Geometry check sheet. Reference: drawing and pictorial views, mm from the part's lowest x, y, z. Round coordinates to 2 decimals unless told otherwise and drop trailing zeros. Loops run counter-clockwise (first coordinate to the right, second up) from the corner with the lowest first, then second, coordinate; pieces in that order, holes last. Notation, with made-up numbers: (45, -17) - (101, -17) arc R22 ccw to (101, 0) - close; hole circle Ø5 at (49.25, 59). An arc over 180 degrees is marked (long way). Return JSON: item names as keys, results as strings.
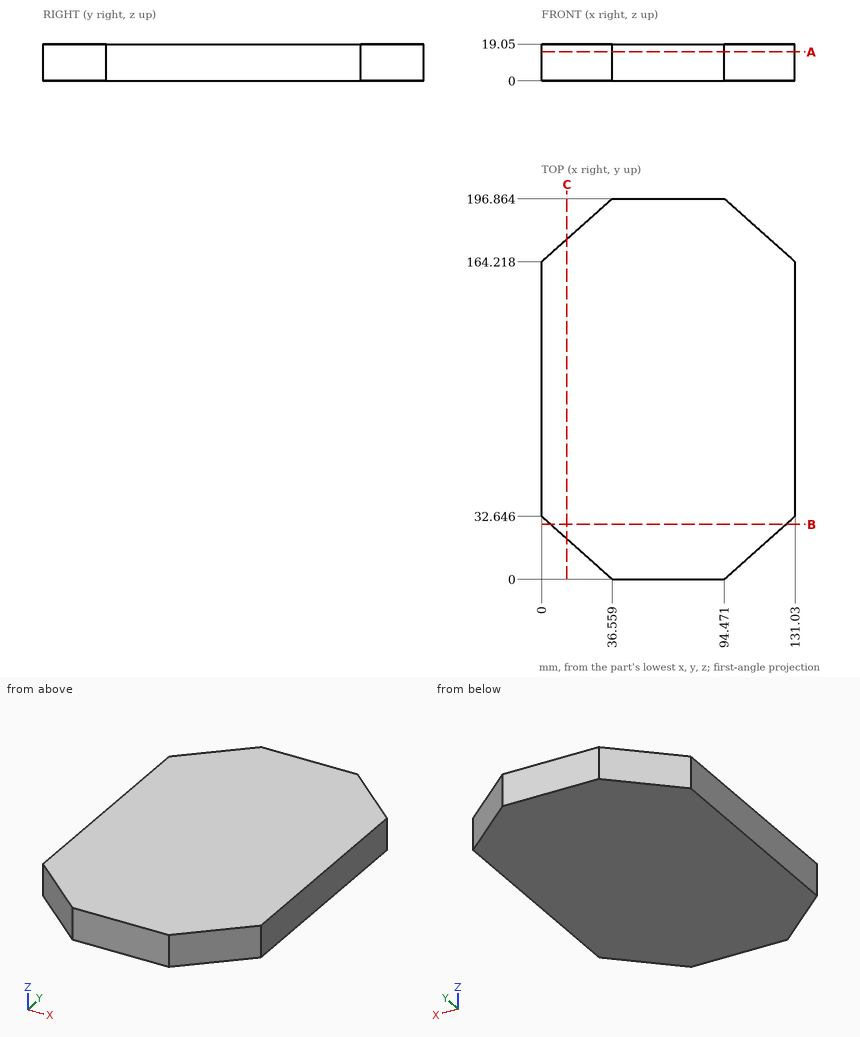
Q1. Scan lines: probe 1 along Y at (x, z) = (101, 10) (1 decimal); probe 2 along X at (y, z) = (170.5, 17) (1 decimal); probe 3 along Y at (x, z) = (107.5, 6.25) (1 decimal). Record each from-to range of solid material in increasing order. Write a range as [from, to].
Answer key:
{"probe 1": "y = [5.8, 191]", "probe 2": "x = [7, 124]", "probe 3": "y = [11.6, 185.2]"}
Q2. Sectioned sample at B-B (y = 28.5). Enter the section's corners in (x, z), plus the area to 3 significant figures.
Answer key:
{"outline": "(4.64, 0) - (126.39, 0) - (126.39, 19.05) - (4.64, 19.05) - close", "area": "2,320 mm²"}
Q3. Sectioned sample at C-C (x = 13). Enter the section's corners in (y, z).
Answer key:
{"outline": "(21.04, 0) - (175.83, 0) - (175.83, 19.05) - (21.04, 19.05) - close"}
Q4. Sectioned sample at A-A (z = 15). Enter the section's corners in (x, y) (1 decimal), plus the area to 3 significant figures.
Answer key:
{"outline": "(0, 32.6) - (36.6, 0) - (94.5, 0) - (131, 32.6) - (131, 164.2) - (94.5, 196.9) - (36.6, 196.9) - (0, 164.2) - close", "area": "23,400 mm²"}
Q5. Depth check by flat-ended pin: P1, Ø6, axis at x = 33.5, z = 10.5, coming from the -Y side; P2, Ø10, axis at x = 111.5, z = 10, coming from the +Y side; P3, Ø5, axis at x = 63.5, y = 35, coming from the -Z side; P4, Ø1, axis at y = 167.5, z = 6.5, coming from the +X side (1 decimal). Enter the tip coordinate at first touch or a pass-through.
Answer key:
{"P1": "stops at y = 0.05", "P2": "stops at y = 186.12", "P3": "stops at z = 0", "P4": "stops at x = 127.9"}
